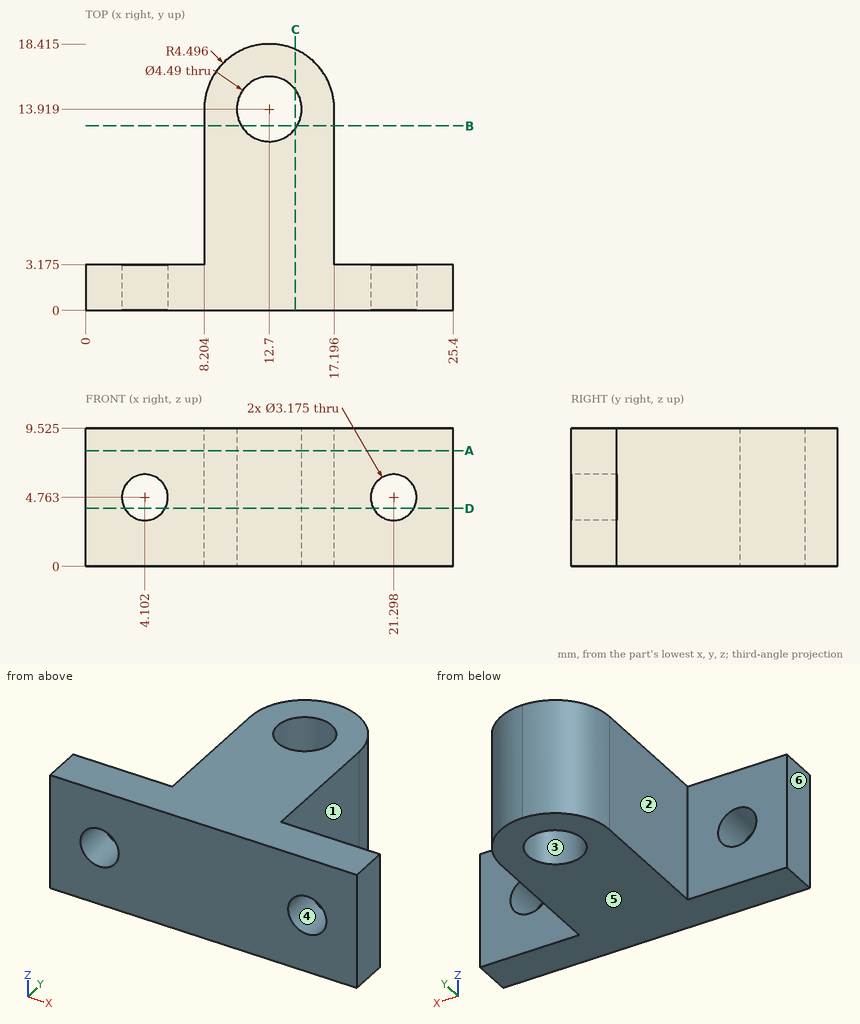
Job drawing, mm, ordinate dimensions from the low corner. One solid piece. A direction names the side the tool comes from. Coordinates: 2 decimals unless noted, no trailing zeros. Write each loop counter-clockwise with the first axis right and the second up, starting at its lowest first coordinate (ties: lowest second). Pieces come first, ordered by that corner, then holes. Notation, with made-up numbers: (28.25, 66.25) - (79.25, 66.25) arc R23 cw to (79.25, 99.25) - close; hole circle Ø11 at (47, 15.25). An arc over 180 degrees is marked (long way). Use a Markdown table: item, result. Add a question column.
Item 1: 3-axis set-ups, long thin cutter, end or side, ignore diameter. For the marked faces 1, 2 and 3: which of +Z, -Z, +X, -X, +Y, -Y reach the whole face in a straight line?
Item 2: Band-saw the part on D-D, the plane z = 4. Give the cut face in (x, y) (1 decimal).
Item 3: Band-saw the part on A-A, the plane z = 8. Give the cut face in (x, y) (1 decimal).
Item 4: Band-saw the part on C-C, the plane x = 14.5. Give the cut face in (y, z) (1 decimal), and give its area (3 significant figures).
Item 5: Drill centre lines: L1, parallel to X at y = 3, z = 4.75 (1 decimal); L2, parallel to X at y = 9.5, z = 8.25 (1 decimal); L3, parallel to Y at x = 6.5, z = 8.25 (1 decimal). Where is each one in solid material? Low to high. Write a range as from..to.
Item 6: Band-saw the part on B-B, the plane y = 12.75. Give the cut face in (x, z) (1 decimal).
Item 7: Flat gauge pins, fed straight in: pin 1 (4 mm diameter, centred on x = 3, z = 6.5, fed in from +Y) (1 decimal); pin 2 (3 mm diameter, centred on y = 11, z = 5.5, fed in from -X). Where does each tip first touch, or does it go through?
Item 8: Mould opens along Z. For the marked faces 4, 5 and 6 say: pulls with the +Z half, pulls with the -Z half, needs draft (parallel to the pull), parting line crosses it, or undercut.
Numbers:
| question | item | result |
|---|---|---|
| 1 | face 1 | +Z, -Z, +X, +Y |
| 1 | face 2 | +Z, -Z, -X, +Y |
| 1 | face 3 | +Z, -Z |
| 2 | outline | (0, 0) - (2.7, 0) - (2.7, 3.2) - (0, 3.2) - close; (5.5, 0) - (19.9, 0) - (19.9, 3.2) - (17.2, 3.2) - (17.2, 13.9) arc R4.5 ccw to (8.2, 13.9) - (8.2, 3.2) - (5.5, 3.2) - close; (22.7, 0) - (25.4, 0) - (25.4, 3.2) - (22.7, 3.2) - close; hole circle Ø4.5 at (12.7, 13.9) |
| 3 | outline | (0, 0) - (25.4, 0) - (25.4, 3.2) - (17.2, 3.2) - (17.2, 13.9) arc R4.5 ccw to (8.2, 13.9) - (8.2, 3.2) - (0, 3.2) - close; hole circle Ø4.5 at (12.7, 13.9) |
| 4 | outline | (0, 0) - (12.6, 0) - (12.6, 9.5) - (0, 9.5) - close; (15.3, 0) - (18, 0) - (18, 9.5) - (15.3, 9.5) - close |
| 4 | area | 146 mm2 |
| 5 | L1 | 0..2.5, 5.7..19.7, 22.9..25.4 |
| 5 | L2 | 8.2..17.2 |
| 5 | L3 | 0..3.2 |
| 6 | outline | (8.2, 0) - (10.8, 0) - (10.8, 9.5) - (8.2, 9.5) - close; (14.6, 0) - (17.2, 0) - (17.2, 9.5) - (14.6, 9.5) - close |
| 7 | pin 1 | y = 3.2 |
| 7 | pin 2 | x = 8.2 |
| 8 | face 4 | undercut |
| 8 | face 5 | pulls with the -Z half |
| 8 | face 6 | needs draft |
